The listing builds one solid part. Answer for the finished solid, in the listing's coordinates (mm). Give positions to 0.01 mm unless a question says otherwise; leave off trailing zeros. Loops run counter-clockwise (first coordinate to the right, second up) from the corner with the lowest first, then second, coordinate; pieces in that order, holes last. Notation, with made-up numbers: (69.5, 27.5) - (121.5, 27.5) arc R16 cw to (121.5, 55.5) - close; hole circle Ø3 at (88, -30.75). An arc over 180 degrees is marked (long way). Answer as CSV lines item,"result". Start each with the question number.
1) A cutting plane is placed at A-A (x = 0). Determine the outline of the cut face in (y, z).
2) A cutting plane is placed at B-B (y = 0). Determine the outline of the cut face in (x, z), and give its area (3 significant figures).
3) A cutting plane is placed at C-C (z = 7). Determine the outline of the cut face in (x, y), and give its area (3 significant figures).
4) Find the intervals of material crossed by line 1 along X through (y, z) = (0, 32); line 2 along Y through (x, z) = (4.5, 11.5); line 3 along Y through (x, z) = (0.25, 20.5), in increasing order.
5) For a pull along Y with two mould halves and no side action, classify faces 1 (the face through (-1.06, 4.773, 19.387)), 2 (the face through (-6, -4, 10.76)), 3 (the face through (-1.495, 6.732, 3.971)) as pulls with the +Y half, pulls with the -Y half, needs draft (parallel to the pull), parting line crosses it, or undercut.
6) A cutting plane is placed at D-D (z = 34.5). Determine the outline of the cut face in (x, y).
7) Flat-ended cylindrical pins translate along their axes: pin 1 (3 mm diameter, centred on y = -1.5, z = 6.5, fed in from -X); pin 2 (3 mm diameter, centred on x = -5, z = 16.5, fed in from -Y); pin 3 (3 mm diameter, centred on y = -5.5, z = 42.5, fed in from +X). Find the tip coordinate at first contact, or state that the pin passes through.
```python
from build123d import *

# Parameters (mm, degrees)
F2_R     = 1.27
F3_R     = 0.508
F4_R     = 2.5527
F5_DEPTH = 12.7
F6_R     = 0.508


with BuildPart() as f1:
    # F0 (on Front) → F1 (revolve)
    with BuildSketch(Plane.XZ):
        Polygon((6.1595, -8.036257), (6.8961, -3.009944), (6.8961, 10.759743), (8.0645, 10.759743), (8.0645, 48.859743), (4.8895, 48.859743), (4.8895, -8.036257), align=None)
    revolve(axis=Axis((0, 0, 17.241214), (0, 0, -1)))

    # F2
    f2_edges = [f1.edges().sort_by_distance(p)[0] for p in [
        (-4.8895, 0, 48.859743),
    ]]
    fillet(f2_edges, radius=F2_R)

    # F3
    f3_edges = [f1.edges().sort_by_distance(p)[0] for p in [
        (-8.0645, 0, 48.859743),
    ]]
    fillet(f3_edges, radius=F3_R)

    # F4 (on Right) → F5 (cut, symmetric)
    with BuildSketch(Plane.YZ):
        with Locations((0, 39.969743)):
            Circle(F4_R)
    extrude(amount=F5_DEPTH, both=True, mode=Mode.SUBTRACT)

    # F6
    f6_edges = [f1.edges().sort_by_distance(p)[0] for p in [
        (-6.1595, 0, -8.036257),
    ]]
    fillet(f6_edges, radius=F6_R)


solid = f1.part
```
Ans:
1,outline,"(-8.06, 10.76) - (-6.9, 10.76) - (-6.9, -3.01) - (-6.22, -7.6) arc R0.51 ccw to (-5.72, -8.04) - (-4.89, -8.04) - (-4.89, 47.59) arc R1.27 ccw to (-6.16, 48.86) - (-7.56, 48.86) arc R0.51 ccw to (-8.06, 48.35) - close; (4.89, -8.04) - (5.72, -8.04) arc R0.51 ccw to (6.22, -7.6) - (6.9, -3.01) - (6.9, 10.76) - (8.06, 10.76) - (8.06, 48.35) arc R0.51 ccw to (7.56, 48.86) - (6.16, 48.86) arc R1.27 ccw to (4.89, 47.59) - close"
2,outline,"(-8.06, 10.76) - (-6.9, 10.76) - (-6.9, -3.01) - (-6.22, -7.6) arc R0.51 ccw to (-5.72, -8.04) - (-4.89, -8.04) - (-4.89, 37.42) - (-8.06, 37.42) - close; (-8.06, 42.52) - (-4.89, 42.52) - (-4.89, 47.59) arc R1.27 ccw to (-6.16, 48.86) - (-7.56, 48.86) arc R0.51 ccw to (-8.06, 48.35) - close; (4.89, -8.04) - (5.72, -8.04) arc R0.51 ccw to (6.22, -7.6) - (6.9, -3.01) - (6.9, 10.76) - (8.06, 10.76) - (8.06, 37.42) - (4.89, 37.42) - close; (4.89, 42.52) - (8.06, 42.52) - (8.06, 48.35) arc R0.51 ccw to (7.56, 48.86) - (6.16, 48.86) arc R1.27 ccw to (4.89, 47.59) - close"
2,area,"280 mm2"
3,outline,"circle Ø13.79 at (0, 0); hole circle Ø9.78 at (0, 0)"
3,area,"74.3 mm2"
4,line 1,"-8.06 to -4.89, 4.89 to 8.06"
4,line 2,"-6.69 to -1.91, 1.91 to 6.69"
4,line 3,"-8.06 to -4.88, 4.88 to 8.06"
5,face 1,"undercut"
5,face 2,"needs draft"
5,face 3,"parting line crosses it"
6,outline,"circle Ø16.13 at (0, 0); hole circle Ø9.78 at (0, 0)"
7,pin 1,"x = -6.9"
7,pin 2,"y = -7.27"
7,pin 3,"x = 7"
